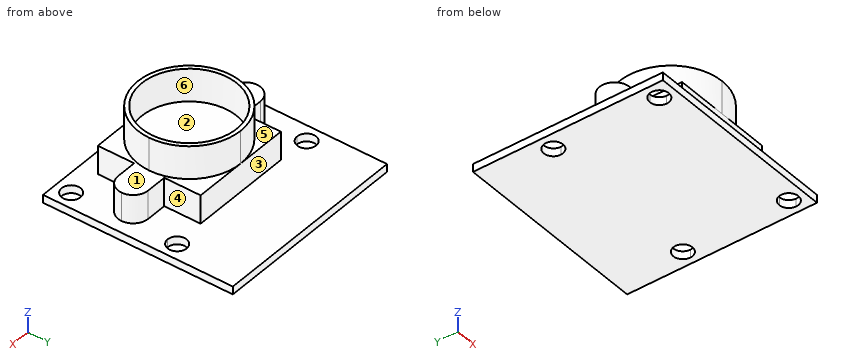
```python
from build123d import *

# Parameters (mm, degrees)
F0_W     = 25
F0_H     = 24
F1_DEPTH = 1
F3_DEPTH = 3.6
F4_R     = 6
F5_DEPTH = 4.16


with BuildPart() as f1:
    # F0 (on Top) → F1 (new body)
    with BuildSketch(Plane.XY):
        Rectangle(F0_W, F0_H)
        with BuildLine():
            ThreePointArc((-9.3, -10), (-11.348528, -10.848528), (-10.5, -8.8))
            ThreePointArc((-10.5, -8.8), (-9.651472, -9.151472), (-9.3, -10))
        make_face(mode=Mode.SUBTRACT)
        with BuildLine():
            ThreePointArc((10.5, -8.8), (11.348528, -9.151472), (11.7, -10))
            ThreePointArc((11.7, -10), (9.651472, -10.848528), (10.5, -8.8))
        make_face(mode=Mode.SUBTRACT)
        with BuildLine():
            ThreePointArc((-10.5, 2.2), (-11.348528, 4.248528), (-9.3, 3.4))
            ThreePointArc((-9.3, 3.4), (-9.651472, 2.551472), (-10.5, 2.2))
        make_face(mode=Mode.SUBTRACT)
        with BuildLine():
            ThreePointArc((11.7, 3.4), (11.348528, 2.551472), (10.5, 2.2))
            ThreePointArc((10.5, 2.2), (9.651472, 4.248528), (11.7, 3.4))
        make_face(mode=Mode.SUBTRACT)
    extrude(amount=F1_DEPTH)

    # F2 (on face) → F3 (join)
    with BuildSketch(Plane.XY.offset(1)):
        Polygon((6.5, 3.25), (-6.5, 3.25), (-6.5, -1.35), (-6.5, -5.15), (-6.5, -9.75), (6.5, -9.75), (6.5, -5.15), (6.5, -1.35), align=None)
        with BuildLine():
            Line((-6.5, -5.15), (-6.5, -1.35))
            Line((-6.5, -1.35), (-9.1, -1.35))
            ThreePointArc((-9.1, -1.35), (-7.756497, -1.906497), (-7.2, -3.25))
            ThreePointArc((-7.2, -3.25), (-7.756497, -4.593503), (-9.1, -5.15))
            Line((-9.1, -5.15), (-6.5, -5.15))
        make_face()
        with BuildLine():
            ThreePointArc((-7.2, -3.25), (-7.756497, -1.906497), (-9.1, -1.35))
            ThreePointArc((-9.1, -1.35), (-11, -3.25), (-9.1, -5.15))
            ThreePointArc((-9.1, -5.15), (-7.756497, -4.593503), (-7.2, -3.25))
        make_face()
        with BuildLine():
            Line((9.1, -1.35), (6.5, -1.35))
            Line((6.5, -1.35), (6.5, -5.15))
            Line((6.5, -5.15), (9.1, -5.15))
            ThreePointArc((9.1, -5.15), (7.2, -3.25), (9.1, -1.35))
        make_face()
        with BuildLine():
            ThreePointArc((11, -3.25), (10.443503, -1.906497), (9.1, -1.35))
            ThreePointArc((9.1, -1.35), (7.2, -3.25), (9.1, -5.15))
            ThreePointArc((9.1, -5.15), (10.443503, -4.593503), (11, -3.25))
        make_face()
    extrude(amount=F3_DEPTH)

    # F4 (on face) → F5 (join)
    with BuildSketch(Plane.XY.offset(4.6)):
        with BuildLine():
            ThreePointArc((0, -9.75), (4.596194, -7.846194), (6.5, -3.25))
            ThreePointArc((6.5, -3.25), (4.596194, 1.346194), (0, 3.25))
            ThreePointArc((0, 3.25), (-6.5, -3.25), (0, -9.75))
        make_face()
        with Locations((0, -3.25)):
            Circle(F4_R, mode=Mode.SUBTRACT)
    extrude(amount=F5_DEPTH)


solid = f1.part
```
The listing builds one solid part. Answer for the finished solid, in the listing's coordinates (mm). Face numbers are marked on the shaded views. A direction names the side the tool comes from. Give positions to 0.01 mm unless a question says otherwise; leave off trailing zeros. Order: outer loops, then holes, each group sorted by start corner. A loop starts at its lowest first (then second) coordinate and runs counter-clockwise, first axis right, second up. Notation, with made-up numbers: (-20, 38) - (29, 38) arc R15 ccw to (29, 55) - close; hole circle Ø10 at (-17, 68). An arc over 180 degrees is marked (long way). Answer in a Markdown table with one row per item. Add a question column.
Q1. The part is cut by section D-D (y = 10). Determine the outline of the cut face in (x, z), then the cut area to 3 significant figures.
Q2. Which of the six approach directions +Z, -Z, +X, -X, +Y, -Y give full straight-line access (tool end or side, diameter ignored) to the marked faces 4, 5 and 6?
Q3. The part is cut by section B-B (x = 2.75). Determine the outline of the cut face in (y, z), then the cut area to 3 significant figures.
Q4. The part is cut by section A-A (z = 2.25). Determine the outline of the cut face in (x, y), then the cut area to 3 significant figures.
Q5. Given P1, Ø2, axis at x = -3.5, z = 6.5, coming from the +Y side; P2, Ø3, axis at y = -7.5, z = 3.5, coming from the +X side; P3, Ø5, axis at y = -9.5, z = 5, coming from the -X side; P4, Ø2, axis at x = 10.5, y = -10, coming from the -Z side, each flat-ended and moving along its own axis, determine where each tip first touches the part or whether it passes through.
Q6. Find the intervals of material crossed by line 1 along Y through (x, z) = (10.5, 0.7); line 2 along X through (y, z) = (3.4, 0.3); line 3 along Y through (x, z) = (-2.25, 2.5), in increasing order. Write a range as [from, to].
Q7. The part is cut by section C-C (z = 6). Determine the outline of the cut face in (x, y).
Q8. For a pull along Y with two mould halves and no side action, classify the marked faces 1, 2 and 3 as released by +Y, released by -Y, zero draft, split by the parting line, or undercut.
Determined:
| question | item | result |
|---|---|---|
| 1 | outline | (-12.5, 0) - (12.5, 0) - (12.5, 1) - (-12.5, 1) - close |
| 1 | area | 25.0 mm² |
| 2 | face 4 | +Z, +X, +Y |
| 2 | face 5 | +Z, -X |
| 2 | face 6 | +Z |
| 3 | outline | (-12, 0) - (12, 0) - (12, 1) - (3.25, 1) - (3.25, 4.6) - (2.64, 4.6) - (2.64, 8.76) - (2.08, 8.76) - (2.08, 4.6) - (-8.58, 4.6) - (-8.58, 8.76) - (-9.14, 8.76) - (-9.14, 4.6) - (-9.75, 4.6) - (-9.75, 1) - (-12, 1) - close |
| 3 | area | 75.4 mm² |
| 4 | outline | (-9.1, -5.15) - (-6.5, -5.15) - (-6.5, -9.75) - (6.5, -9.75) - (6.5, -5.15) - (9.1, -5.15) arc R1.9 ccw to (9.1, -1.35) - (6.5, -1.35) - (6.5, 3.25) - (-6.5, 3.25) - (-6.5, -1.35) - (-9.1, -1.35) arc R1.9 ccw to start |
| 4 | area | 200 mm² |
| 5 | P1 | stops at y = 2.75 |
| 5 | P2 | stops at x = 6.5 |
| 5 | P3 | stops at x = -6.5 |
| 5 | P4 | passes through |
| 6 | line 1 | y = [-12, -11.2], [-8.8, 2.2], [4.6, 12] |
| 6 | line 2 | x = [-12.5, -11.7], [-9.3, 9.3], [11.7, 12.5] |
| 6 | line 3 | y = [-9.75, 3.25] |
| 7 | outline | circle Ø13 at (0, -3.25); hole circle Ø12 at (0, -3.25) |
| 8 | face 1 | zero draft |
| 8 | face 2 | undercut |
| 8 | face 3 | released by +Y |
